Here's how the part is built. I have some questions about the finished solid (model axes, mm). Coordinates: 2 decimals unless noted, no trailing zeros. Write each loop counter-clockwise with the first axis right and the second up, starting at its lowest first coordinate (ties: lowest second). Pieces come first, ordered by that corner, then holes. Notation, with made-up numbers: M 21.25,-36.75 L 38.25,-36.75 A16 ccw 38.25,-15.75 Z; hole C 6,44 d7. An arc over 180 degrees is marked long. Use a Markdown table: item, result.
```python
from build123d import *

# Parameters (mm, degrees)
BOSS_EXTRUDE1_DEPTH             = 3
SKETCH5_W                       = 3
SKETCH5_H                       = 10
CUT_EXTRUDE2_DEPTH              = 100.040395799
CIRPATTERN1_COUNT               = 5
CIRPATTERN1_ANGLE               = 80
CIRPATTERN1_THE_OTHER_WAY_COUNT = 5
CIRPATTERN1_THE_OTHER_WAY_ANGLE = 80
SKETCH6_R                       = 18
CUT_EXTRUDE3_DEPTH              = 100.029036146


with BuildPart() as part:
    # Sketch4 → Boss-Extrude1 (new body)
    with BuildSketch(Plane.XY):
        with BuildLine():
            Line((70, 0), (-70, 0))
            ThreePointArc((-70, 0), (0, -70), (70, 0))
        make_face()
    extrude(amount=BOSS_EXTRUDE1_DEPTH)

    # Sketch5 → Cut-Extrude2 (cut, through all)
    with BuildSketch(Plane.XY):
        with Locations((0, -65)):
            Rectangle(SKETCH5_W, SKETCH5_H)
    cut_extrude2 = extrude(amount=CUT_EXTRUDE2_DEPTH, mode=Mode.SUBTRACT)

    # CirPattern1: Cut-Extrude2 ×5 about axis
    cirpattern1_axis = Axis((0, 0, 0), (0, 0, -1))
    for i in range(1, CIRPATTERN1_COUNT):
        add(cut_extrude2.rotate(cirpattern1_axis, i * CIRPATTERN1_ANGLE / (CIRPATTERN1_COUNT - 1)), mode=Mode.SUBTRACT)

    # CirPattern1 the other way: Cut-Extrude2 ×5 about axis
    cirpattern1_the_other_way_axis = Axis((0, 0, 0), (0, 0, 1))
    for i in range(1, CIRPATTERN1_THE_OTHER_WAY_COUNT):
        add(cut_extrude2.rotate(cirpattern1_the_other_way_axis, i * CIRPATTERN1_THE_OTHER_WAY_ANGLE / (CIRPATTERN1_THE_OTHER_WAY_COUNT - 1)), mode=Mode.SUBTRACT)

    # Sketch6 → Cut-Extrude3 (cut, through all)
    with BuildSketch(Plane.XY):
        Circle(SKETCH6_R)
    extrude(amount=CUT_EXTRUDE3_DEPTH, mode=Mode.SUBTRACT)


solid = part.part
```
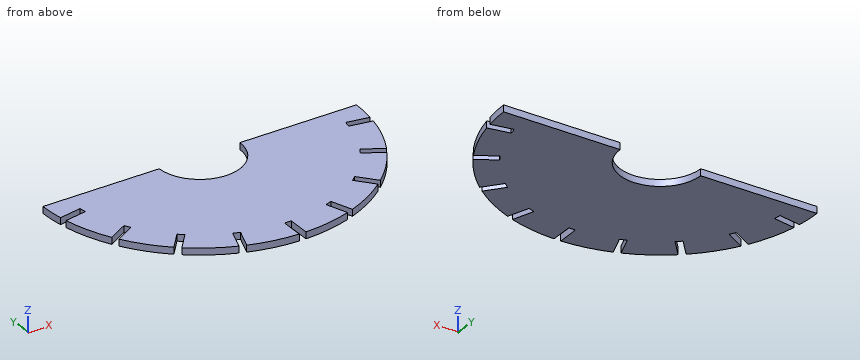
1. Suppose I cut it at B-B on y = -25.5. Write out the boundary of the cut face in (x, z), and give its area (3 significant figures).
Answers follow:
| item | result |
|---|---|
| outline | M -65.19,0 L 65.19,0 L 65.19,3 L -65.19,3 Z |
| area | 391 mm2 |
2. Will these pins go through, and if not, where does the flat tip stop? pin 1 Ø1 at (x, z) = (22.5, 1.5) entering from -Y; pin 2 Ø1 at (y, z) = (-20.5, 0.5) entering from -X; pin 3 Ø1.5 at (x, z) = (0, 1) entering from -Y.
Answers follow:
| item | result |
|---|---|
| pin 1 | stops at y = -66.45 |
| pin 2 | stops at x = -67.08 |
| pin 3 | stops at y = -60 |
3. I need wall thicknesses on probe 1 along X at (y, z) = (-65, 1.65); probe 2 along X at (y, z) = (-3, 2.35); probe 3 along X at (y, z) = (-57.5, 1). Which ranges of each line are inside material? Lowest first, please.
Answers follow:
| item | result |
|---|---|
| probe 1 | x = -25.98 to -25.25, -22.06 to -1.5, 1.5 to 22.06, 25.25 to 25.98 |
| probe 2 | x = -69.94 to -17.75, 17.75 to 69.94 |
| probe 3 | x = -39.92 to -22.52, -19.33 to 19.33, 22.52 to 39.92 |
4. Suppose I cut it at A-A on x = 0. Write out the boundary of the cut face in (y, z).
Answers follow:
| item | result |
|---|---|
| outline | M -60,0 L -18,0 L -18,3 L -60,3 Z |
